Input: part model. Units: mm. Frame: model coordinates. A direction names the side the tool comes from. Coordinates: 2 decimals unless noted, no trailing zeros. Write each loop counter-clockwise with the first axis right and the second up, starting at its lowest first coordinate (ties: lowest second). Pieces come first, ordered by that corner, then holes.
1) Pin query (flat end, axial travel): pin 1 Ø7 at (x, y) = (26.5, -14.5) entering from -Z; pin 2 Ø6 at (x, y) = (11.5, 35.5) entering from -Z; pin 3 Ø8 at (x, y) = (13.5, 10.5) entering from +Z; pin 4 Ø10 at (y, z) = (-8.5, -1) entering from -X. Return the tip coordinate at first contact, or that it passes through.
2) Line query: L1, parallel to Z at x = 29, y = -11; L2, parallel to X at y = 13.5, z = -5.5; L3, parallel to X at y = 6.5, z = 8.5. Output: solid intervals per line, ascending.
3) Draft query along Y for faces 1 (the cylindrical face through (30, 19.16, -3.02)), 2 (the cylindrical face through (6.805, 39.603, 7.946)), 3 (the flat face through (22.542, 7.355, -9.347)), 4 (the flat face through (26, -9, 26.632)). Return one class per face: pulls with the +Y half, pulls with the -Y half, needs draft (parallel to the pull), parting line crosses it, or undercut.
4) Section query C-C (z = 12). Output: boundary loops of the cut face in (x, y).
5) Set-up query: faces 5 (the flat face through (26, 5.016, 13)), 6 (the flat face through (26, 6.616, 9)), 7 (the flat face through (19.05, 5.2, 8.1)). Return all of +Z, -Z, +X, -X, +Y, -Y with unobstructed straight access to the full face (end or side cutting, diameter ignored); none if empty.
6) Section query A-A (y = -3). Output: boundary loops of the cut face in (x, z), then the cut area to 3 significant figures.
7) Section query D-D (y = 13). Output: boundary loops of the cut face in (x, z), then the cut area to 3 significant figures.
Autodesk Inventor part; units mm, degrees
ref_plane "YZ Plane" through (0, 0, 0) normal (1, 0, 0) x (0, 1, 0)
ref_plane "XZ Plane" through (0, 0, 0) normal (0, 1, 0) x (-1, 0, 0)
ref_plane "XY Plane" through (0, 0, 0) normal (0, 0, 1) x (1, 0, 0)
sketch "Sketch1" plane through (0, 0, 0) normal (1, 0, 0) x (0, 1, 0)
  line L0 (6.6158, 26.6317) -> (-24.673, 26.6317)
  line L1 (6.6158, 0.5934) -> (6.6158, 26.6317)
  line L2 (5.0158, 25.0317) -> (-24.673, 25.0317)
  line L3 (-24.673, 1.8624) -> (5.0158, 1.8624)
  line L4 (5.0158, 1.8624) -> (5.0158, 25.0317)
  line L5 (-24.673, 26.6317) -> (-24.673, 25.0317)
  line L6 (-24.673, 1.8624) -> (-24.673, 0.1625)
  line L7 (-24.6286, 24.997) -> (4.9714, 24.997) construction
  line L8 (4.9714, 24.997) -> (4.9714, 1.897) construction
  line L9 (4.9714, 1.897) -> (-24.6286, 1.897) construction
  line L10 (-24.6286, 1.897) -> (-24.6286, 24.997) construction
  line L11 (-24.6286, 1.897) -> (-24.6286, 1.8624) construction
  line L12 (-24.6286, 24.997) -> (-24.6286, 25.0317) construction
  line L13 (4.9714, 2.1686) -> (16.2714, -18.903) construction
  line L14 (4.0247, -13.8964) -> (20.8987, -4.8474)
  line L15 (3.4408, -13.2733) -> (44.9775, 9.0015)
  line L16 (3.4408, -13.2733) -> (3.4408, 0.1625)
  line L17 (6.6158, 0.5934) -> (6.6158, -7.968)
  line L18 (6.6158, -7.968) -> (43.477, 11.7995)
  line L19 (43.477, 11.7995) -> (44.9775, 9.0015)
  line L20 (-24.673, 0.1625) -> (3.4408, 0.1625)
  line L21 (6.6158, 13.8186) -> (15.6898, -3.1019) construction
  point P0 (0, 0)
  dimension "d2" = 1.6
  dimension "d3" = 23.1693
  dimension "d5" = 29.6888
  dimension "d6" = 29.6
  dimension "d7" = 23.1
  dimension "d8" = 0.0444
  dimension "d9" = 11.3
  dimension "d10" = 20.8
  dimension "d11" = 10.2
  dimension "d15" = 3.175
  dimension "d22" = 4
  dimension "d23" = 3.175
  dimension "d28" = 19.2
extrude "Extrusion1" add sketch "Sketch1" along normal blind 32.6644
sketch "Sketch2" plane through (0, 6.6158, -7.968) normal (0, -0.4726007, 0.8812767) x (1, 0, 0)
  circle A0 centre (17.209, 24.6192) radius 16.4
  circle A1 centre (28.8056, 13.0227) radius 1.25
  circle A2 centre (5.6125, 36.2158) radius 1.25
  line L0 (28.8056, 13.0227) -> (5.6125, 36.2158) construction
  line L1 (0, 41.827) -> (32.6644, 41.827)
  line L2 (0, 3.3414) -> (38.1, 3.3414) construction
  line L3 (0, 41.827) -> (0, 0) construction
  circle A3 centre (11.5522, 18.9624) radius 1.4362 construction
  line L4 (11.5522, 18.9624) -> (17.209, 24.6192) construction
  line L5 (0, 10.2963) -> (32.6644, 10.2963) construction
  line L6 (32.6644, 41.827) -> (32.6644, 0) construction
  circle A4 centre (17.209, 24.6192) radius 13.95 construction
  line L7 (28.8056, 13.0227) -> (5.6125, 36.2158) construction
  line L8 (31.7345, 15.4934) -> (8.3123, 38.9155)
  line L9 (2.9127, 33.516) -> (26.1058, 10.3229)
  arc A5 (26.1058, 10.3229) -> (26.1326, 10.2963) centre (28.8056, 13.0227) ccw
  arc A6 (8.3123, 38.9155) -> (2.9127, 33.516) centre (5.6125, 36.2158) ccw
  line L10 (32.6644, 13.2483) -> (32.6644, 0)
  line L11 (0, 0) -> (32.6644, 0)
  line L12 (26.1326, 10.2963) -> (26.1326, 0)
  arc A7 (32.6644, 13.2483) -> (31.7345, 15.4934) centre (29.4894, 13.2483) ccw
  line L13 (0, 0) -> (0, 41.827)
  line L14 (32.6644, -5.3054) -> (32.6644, 41.827)
  arc A8 (17.872, 18.5567) -> (11.1465, 25.2822) centre (11.4175, 18.8277) ccw
  point P0 (0, -2.0647)
  point P1 (0, 3.3414)
  point P2 (0, 10.2963)
  point P3 (31.1867, 16.0411)
  point P4 (32.6644, 19.1336)
  point P5 (32.6644, 13.2483)
  point P6 (15.9856, 23.3958)
  dimension "d16" = 32.8
  dimension "d17" = 2.5
  dimension "d18" = 2.5
  dimension "d19" = 45
  dimension "d26" = 8
  dimension "d27" = 15.621
  dimension "d29" = 27.9
  dimension "d30" = 3.175
extrude "Extrusion2" cut sketch "Sketch2" against normal blind 25.4 contours A2 A0 | A0 A2 | A1 A0 | A0 A1
extrude "Extrusion3" cut sketch "Sketch2" against normal blind 25.4 contours L14 A0 L8 | A0 L8 A6 L9 A5 L12 L11 L13 L1 L14 | L14 A7 L8 A0 | L9 A0 | A8 L9
sketch "Sketch5" plane through (0, 0, 0) normal (-1, 0, 0) x (0, 0, 1)
  line L0 (-7.968, 6.6158) -> (-10.766, 8.1163)
  line L1 (-13.2733, 3.4408) -> (-10.766, 8.1163)
  line L2 (0.1625, 3.4408) -> (-13.2733, 3.4408)
  line L3 (0.1625, -24.673) -> (0.1625, 3.4408)
  line L4 (1.8624, -24.673) -> (0.1625, -24.673)
  line L5 (1.8624, 5.0158) -> (1.8624, -24.673)
  line L6 (25.0317, 5.0158) -> (1.8624, 5.0158)
  line L7 (25.0317, -24.673) -> (25.0317, 5.0158)
  line L8 (26.6317, -24.673) -> (25.0317, -24.673)
  line L9 (26.6317, 6.6158) -> (26.6317, -24.673)
  line L10 (-7.968, 6.6158) -> (26.6317, 6.6158)
  point P0 (0, 0)
extrude "Extrusion4" cut sketch "Sketch5" against normal blind 19.05
properties part number "Motor Mount"
Answer:
1. pin 1: stops at z = 0.16
1. pin 2: stops at z = 2.31
1. pin 3: passes through
1. pin 4: stops at x = 19.05
2. L1: z = 0.16 to 1.86, 25.03 to 26.63
2. L2: x = 26.13 to 32.66
2. L3: x = 19.05 to 32.66
3. face 1: undercut
3. face 2: undercut
3. face 3: pulls with the +Y half
3. face 4: needs draft
4. outline: (19.05, 5.02) - (32.66, 5.02) - (32.66, 6.62) - (19.05, 6.62) - close
5. face 5: +X, -X, -Y
5. face 6: +Z, +X, -X
5. face 7: +Z, -Z, -X, -Y
6. outline: (19.05, 0.16) - (32.66, 0.16) - (32.66, 1.86) - (19.05, 1.86) - close; (19.05, 25.03) - (32.66, 25.03) - (32.66, 26.63) - (19.05, 26.63) - close
6. area: 44.9 mm2
7. outline: (26.13, -8.15) - (32.66, -8.15) - (32.66, -4.54) - (26.13, -4.54) - close
7. area: 23.5 mm2
